Geometry: final body of the model. Coordinates: model frame, mm. Coordinates: 2 decimals unless noted, no trailing zeros. Loops run counter-clockwise (first coordinate to the right, second up) from the corner with the lowest first, then second, coordinate; pieces in that order, holes last. Notation, with made-up numbers: (-19.75, 64) -> (-8.75, 64) arc R19 ccw to (-8.75, 86) -> close; hole circle Ø2 at (-20.5, -0.5). An arc over 180 degrees is marked (long way). One line per item, written item: value. Start each with the question number.
Autodesk Inventor part; units mm, degrees
ref_plane "YZ Plane" through (0, 0, 0) normal (1, 0, 0) x (0, 1, 0)
ref_plane "XZ Plane" through (0, 0, 0) normal (0, 1, 0) x (-1, 0, 0)
ref_plane "XY Plane" through (0, 0, 0) normal (0, 0, 1) x (1, 0, 0)
sketch "Sketch1" plane through (0, 0, 0) normal (0, 1, 0) x (-1, 0, 0)
  line L0 (14.7043, 12.4547) -> (0.2043, 12.4547)
  line L1 (0.2043, 12.4547) -> (0.2043, -0.5453)
  line L2 (0.2043, -0.5453) -> (14.7043, -0.5453)
  line L3 (14.7043, -0.5453) -> (14.7043, 12.4547)
  line L4 (14.7043, 12.4547) -> (0.2043, -0.5453) construction
  line L5 (0.2043, 12.4547) -> (14.7043, -0.5453) construction
  point P0 (0, 0)
  point P1 (7.4543, 5.9547)
  dimension "d0" = 14.5
  dimension "d1" = 13
extrude "Extrusion1" add sketch "Sketch1" along normal blind 3
sketch "Sketch2" plane through (0, 3, 0) normal (0, 1, 0) x (1, 0, 0)
  circle A0 centre (-7.7043, -10.4547) radius 1
  circle A1 centre (-7.7043, -1.4547) radius 1
  line L0 (-14.7043, -12.4547) -> (-0.2043, -12.4547)
  line L1 (-14.7043, 0.5453) -> (-14.7043, -12.4547)
  line L2 (-0.2043, 0.5453) -> (-14.7043, 0.5453)
  point P0 (0, 0)
  dimension "d4" = 2
  dimension "d5" = 2
  dimension "d6" = 2
  dimension "d7" = 7
  dimension "d8" = 7
  dimension "d9" = 2
extrude "Extrusion2" cut sketch "Sketch2" against normal blind 3
properties part number "USB holder"
1. Section B-B on x = -7. Return the cut outline in (y, z), plus the area to 3 significant figures.
2. Draft query along Z for faces 1 (the face through (-8.703, 1.521, 1.411)), 2 (the face through (-8.703, 1.521, 10.411)), 3 (the face through (-7, 1, -0.545)), 4 (the face through (-7, 3, 6)). Return one class per face: released by +Z, released by -Z, zero draft, split by the parting line, or undercut.
3. Line query: L1, parallel to Z at x = -8.5, y = 2.2; L2, parallel to X at y = 1.2, z = 10.5; L3, parallel to X at y = 1.45, z = 10. Output: solid intervals per line, ascending. Write a range as [from, to].
4. Section C-C on y = 0.85. Return the cut outline in (x, z), plus the area to 3 significant figures.
5. Section A-A on z = 10. Return the cut outline in (x, y).
6. Section D-D on z = 1.75. Return the cut outline in (x, y).
Checks:
1. outline: (0, -0.55) -> (3, -0.55) -> (3, 0.74) -> (0, 0.74) -> close; (0, 2.16) -> (3, 2.16) -> (3, 9.74) -> (0, 9.74) -> close; (0, 11.16) -> (3, 11.16) -> (3, 12.45) -> (0, 12.45) -> close
1. area: 30.5 mm²
2. face 1: undercut
2. face 2: undercut
2. face 3: released by -Z
2. face 4: zero draft
3. L1: [-0.55, 0.85], [2.06, 9.85], [11.06, 12.45]
3. L2: [-14.7, -8.7], [-6.71, -0.2]
3. L3: [-14.7, -8.59], [-6.81, -0.2]
4. outline: (-14.7, -0.55) -> (-0.2, -0.55) -> (-0.2, 12.45) -> (-14.7, 12.45) -> close; hole circle Ø2 at (-7.7, 1.45); hole circle Ø2 at (-7.7, 10.45)
4. area: 182 mm²
5. outline: (-14.7, 0) -> (-8.59, 0) -> (-8.59, 3) -> (-14.7, 3) -> close; (-6.81, 0) -> (-0.2, 0) -> (-0.2, 3) -> (-6.81, 3) -> close
6. outline: (-14.7, 0) -> (-8.66, 0) -> (-8.66, 3) -> (-14.7, 3) -> close; (-6.75, 0) -> (-0.2, 0) -> (-0.2, 3) -> (-6.75, 3) -> close
